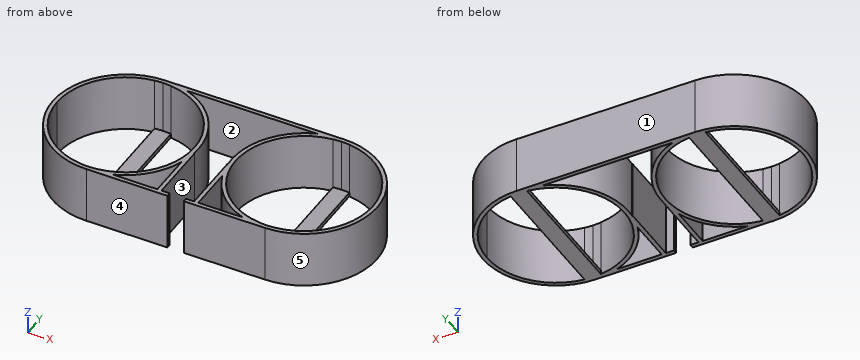
```python
from build123d import *

# Parameters (mm, degrees)
F0_W     = 5
F0_H     = 2.5
F0_W_2   = 2.5
F1_DEPTH = 35
F2_DEPTH = 2.5


with BuildPart() as f1:
    # F0 (on Top) → F1 (new body)
    with BuildSketch(Plane.XY):
        with Locations((7.5, 1.25)):
            Rectangle(F0_W, F0_H)
        with Locations((11.25, 1.25)):
            Rectangle(F0_W_2, F0_H)
        with BuildLine():
            Line((10, 40), (10, 2.5))
            Line((10, 2.5), (12.5, 2.5))
            Line((12.5, 2.5), (12.5, 29.7945588301))
            ThreePointArc((12.5, 29.7945588301), (11.0632944452, 34.8303252101), (10.2281127576, 40))
            Line((10.2281127576, 40), (10, 40))
        make_face()
        with BuildLine():
            Line((12.5, 2.5), (12.5, 0))
            Line((12.5, 0), (54.5, 0))
            ThreePointArc((54.5, 0), (47.0417830549, 0.6294517928), (39.7945588301, 2.5))
            Line((39.7945588301, 2.5), (12.5, 2.5))
        make_face()
        with BuildLine():
            Line((39.7945588301, 2.5), (54.5, 2.5))
            ThreePointArc((54.5, 2.5), (51.9955434529, 2.574736764), (49.5, 2.798681076))
            ThreePointArc((49.5, 2.798681076), (12.5, 44.5), (49.5, 86.201318924))
            ThreePointArc((49.5, 86.201318924), (51.9955434529, 86.425263236), (54.5, 86.5))
            Line((54.5, 86.5), (39.7945588301, 86.5))
            ThreePointArc((39.7945588301, 86.5), (16.948118334, 68.3768964344), (10.2281127576, 40))
            Line((10.2281127576, 40), (12.5, 40))
            Line((12.5, 40), (12.5, 29.7945588301))
            ThreePointArc((12.5, 29.7945588301), (23.0337482372, 13.0337482372), (39.7945588301, 2.5))
        make_face()
        with BuildLine():
            ThreePointArc((10.2281127576, 40), (11.0632944452, 34.8303252101), (12.5, 29.7945588301))
            Line((12.5, 29.7945588301), (12.5, 40))
            Line((12.5, 40), (10.2281127576, 40))
        make_face()
        with BuildLine():
            ThreePointArc((39.7945588301, 2.5), (47.0417830549, 0.6294517928), (54.5, 0))
            Line((54.5, 0), (54.5, 2.5))
            Line((54.5, 2.5), (39.7945588301, 2.5))
        make_face()
        with BuildLine():
            Line((54.5, 2.5), (54.5, 0))
            ThreePointArc((54.5, 0), (85.9662517628, 13.0337482372), (99, 44.5))
            ThreePointArc((99, 44.5), (85.9662517628, 75.9662517628), (54.5, 89))
            Line((54.5, 89), (54.5, 86.5))
            ThreePointArc((54.5, 86.5), (57.0044565471, 86.425263236), (59.5, 86.201318924))
            ThreePointArc((59.5, 86.201318924), (85.9165561448, 72.3747197295), (96.5, 44.5))
            ThreePointArc((96.5, 44.5), (85.9165561448, 16.6252802705), (59.5, 2.798681076))
            ThreePointArc((59.5, 2.798681076), (57.0044565471, 2.574736764), (54.5, 2.5))
        make_face()
        with BuildLine():
            Line((54.5, 86.5), (54.5, 89))
            ThreePointArc((54.5, 89), (47.0417830549, 88.3705482072), (39.7945588301, 86.5))
            Line((39.7945588301, 86.5), (54.5, 86.5))
        make_face()
        with BuildLine():
            ThreePointArc((39.7945588301, 86.5), (47.0417830549, 88.3705482072), (54.5, 89))
            Line((54.5, 89), (0, 89))
            Line((0, 89), (0, 86.5))
            Line((0, 86.5), (39.7945588301, 86.5))
        make_face()
    extrude(amount=F1_DEPTH)

    # F0 (on Top) → F2 (join)
    with BuildSketch(Plane.XY):
        with BuildLine():
            Line((54.5, 86.5), (54.5, 44.5))
            Line((54.5, 44.5), (59.5, 44.5))
            Line((59.5, 44.5), (59.5, 86.201318924))
            ThreePointArc((59.5, 86.201318924), (57.0044565471, 86.425263236), (54.5, 86.5))
        make_face()
        with BuildLine():
            Line((49.5, 44.5), (54.5, 44.5))
            Line((54.5, 44.5), (54.5, 86.5))
            ThreePointArc((54.5, 86.5), (51.9955434529, 86.425263236), (49.5, 86.201318924))
            Line((49.5, 86.201318924), (49.5, 44.5))
        make_face()
        with BuildLine():
            ThreePointArc((49.5, 2.798681076), (51.9955434529, 2.574736764), (54.5, 2.5))
            Line((54.5, 2.5), (54.5, 44.5))
            Line((54.5, 44.5), (49.5, 44.5))
            Line((49.5, 44.5), (49.5, 2.798681076))
        make_face()
        with BuildLine():
            Line((54.5, 44.5), (54.5, 2.5))
            ThreePointArc((54.5, 2.5), (57.0044565471, 2.574736764), (59.5, 2.798681076))
            Line((59.5, 2.798681076), (59.5, 44.5))
            Line((59.5, 44.5), (54.5, 44.5))
        make_face()
    extrude(amount=F2_DEPTH)

    # F3: F1 across plane


with BuildPart() as f1_1:
    add(f1.part)
    add(f1.part.mirror(Plane.YZ))


solid = f1_1.part
```
Work out the finished part from the listing and answer in its coordinate system (mm). Face numbers are marked on the shaded views. A direction names the side the tool comes from. Round coordinates to 2 decimals unless told otherwise and drop trailing zeros. Order: outer loops, then holes, each group sorted by start corner. A loop starts at its lowest first (then second) coordinate and runs counter-clockwise, first axis right, second up.
Q1. A cutting plane is placed at D-D, the plane x = -25.5. Determine the outline of the cut face in (y, z).
Solution:
outline: (0, 0) - (2.5, 0) - (2.5, 35) - (0, 35) - close; (10.75, 0) - (14.12, 0) - (14.12, 35) - (10.75, 35) - close; (74.88, 0) - (78.25, 0) - (78.25, 35) - (74.88, 35) - close; (86.5, 0) - (89, 0) - (89, 35) - (86.5, 35) - close
Q2. Find the intervals of material crossed by line 1 along X through (y, z) = (20.5, 5); line 2 along X through (y, z) = (34, 9.5); line 3 along X through (y, z) = (8, 15.5), in increasing order.
Solution:
line 1: x = -91.97 to -88.97, -20.03 to -17.03, -12.5 to -10, 10 to 12.5, 17.03 to 20.03, 88.97 to 91.97
line 2: x = -97.74 to -95.17, -13.83 to -10, 10 to 13.83, 95.17 to 97.74
line 3: x = -79.96 to -75.28, -33.72 to -29.04, -12.5 to -10, 10 to 12.5, 29.04 to 33.72, 75.28 to 79.96
Q3. A cutting plane is placed at B-B, the plane y = 83. Determine the outline of the cut face in (x, z), then the cut area to 3 significant figures.
Solution:
outline: (-76.82, 0) - (-71.29, 0) - (-71.29, 35) - (-76.82, 35) - close; (-59.5, 0) - (-49.5, 0) - (-49.5, 2.5) - (-59.5, 2.5) - close; (-37.71, 0) - (-32.18, 0) - (-32.18, 35) - (-37.71, 35) - close; (32.18, 0) - (37.71, 0) - (37.71, 35) - (32.18, 35) - close; (49.5, 0) - (59.5, 0) - (59.5, 2.5) - (49.5, 2.5) - close; (71.29, 0) - (76.82, 0) - (76.82, 35) - (71.29, 35) - close
area: 824 mm2
Q4. Given pin 1 Ø11 at (x, y) = (53.5, 24.5) entering from +Z; pin 2 Ø13.5 at (y, z) = (15.5, 21.5) entering from -X; pin 3 Ø3 at (y, z) = (32, 0.5) entering from -X, each flat-ended and moving along its own axis, determine where each tip first touches the part or whether it passes through.
Solution:
pin 1: stops at z = 2.5
pin 2: stops at x = -93.04
pin 3: stops at x = -97.62
Q5. The mould has two halves that part along X. Classify the marked faces 3, 4 and 5: pulls with the +X half, pulls with the -X half, needs draft (parallel to the pull), parting line crosses it, or undercut.
Solution:
face 3: undercut
face 4: needs draft
face 5: pulls with the +X half
Q6. A cutting plane is placed at A-A, the plane x = 16. Determine the outline of the cut face in (y, z), then the cut area to 3 significant figures.
Solution:
outline: (0, 0) - (2.5, 0) - (2.5, 35) - (0, 35) - close; (22.18, 0) - (27.71, 0) - (27.71, 35) - (22.18, 35) - close; (61.29, 0) - (66.82, 0) - (66.82, 35) - (61.29, 35) - close; (86.5, 0) - (89, 0) - (89, 35) - (86.5, 35) - close
area: 562 mm2
Q7. A tool of negligible diameter and unlimited length cuts with its end or side. For the marked faces 1 and 2, from which of +Z, -Z, +X, -X, +Y, -Y can it reach the whole face along a straight path? Write none if from no direction.
Solution:
face 1: +Z, -Z, +X, -X, +Y
face 2: +Z, -Z
Q8. A cutting plane is placed at C-C, the plane z = 6.5. Determine the outline of the cut face in (x, y).
Solution:
outline: (-54.5, 0) - (-5, 0) - (-5, 2.5) - (-10, 2.5) - (-10, 40) - (-10.23, 40) arc R44.5 ccw to (-39.79, 86.5) - (39.79, 86.5) arc R44.5 ccw to (10.23, 40) - (10, 40) - (10, 2.5) - (5, 2.5) - (5, 0) - (54.5, 0) arc R44.5 ccw to (54.5, 89) - (-54.5, 89) arc R44.5 ccw to start; hole circle Ø84 at (-54.5, 44.5); hole (-39.79, 2.5) - (-12.5, 2.5) - (-12.5, 29.79) arc R44.5 cw to start; hole (12.5, 2.5) - (39.79, 2.5) arc R44.5 cw to (12.5, 29.79) - close; hole circle Ø84 at (54.5, 44.5)
